Work out the finished part from the listing and answer in its coordinate system (mm). A direction names the side the tool comes from. Coordinates: 2 decimals unless noted, no trailing zeros. Order: outer loops, then holes, each group sorted by start corner. A loop starts at its lowest first (then second) coordinate and runs counter-clockwise, first axis right, second up. Notation, with made-up numbers: (82.5, -3) - (89.5, -3) arc R6 ccw to (89.5, 2) - close; hole circle Ø7 at (73, 37.25). An arc over 180 degrees is marked (long way). Answer as a JSON object with one key per item and string values. Group by question number.
1) Section B-B (y = 5) is taken. Give the vertices of the cut face in (x, z), plus the area to 3 significant figures.
2) Find the intervals of material crossed by line 1 along Z through (x, y) = (-10.45, 1.55); line 2 along X through (y, z) = (2.05, 5.2); line 3 along Z through (x, y) = (12.95, 2.55), in increasing order.
3) Section C-C (z = 5.2) is taken. Give the vertices of the cut face in (x, y).
4) Section A-A (x = -2.5) is taken. Give the vertices of the cut face in (y, z), plus the area to 3 significant figures.
5) The mould has two halves that part along Y. Classify faces 1 (the face through (1, 13, 14)), 2 (the face through (1, 9, -15)), 3 (the face through (-16.25, 1, 0)), 4 (the face through (-5.035, 5.535, 7.501)): released by +Y, released by -Y, zero draft, split by the parting line, or undercut.
6) Each of these flat-tipped pins is pushed along its axis until it touches: P1, Ø5, axis at x = -1, z = -14, coming from the -Y side; P2, Ø3.5, axis at x = -10.45, z = 15.6, coming from the +Y side; P3, Ø6, axis at x = -12.5, z = -1.5, coming from the +Y side. Where does it stop, or does it pass through?
7) Section D-D (y = 12) is taken. Give the vertices of the cut face in (x, z).
8) A tool of negligible diameter and unlimited length cuts with its end or side. For faces 5 (the face through (7.535, 5.465, 7.501)), 6 (the face through (6.965, 8.699, 14.69)), 7 (the face through (13.258, 2.081, -14.132)), 8 (the face through (1.32, 9.301, -7.485)), from which of +Z, -Z, +X, -X, +Y, -Y can it reach the whole face along a straight path? Write none if from no direction.
from build123d import *

# Parameters (mm, degrees)
SKETCH_2_W             = 32.5
SKETCH_2_H             = 42
SKETCH_2_R             = 1.5
SKETCH_2_R_2           = 1.449840903
EXTRUDE_1_DEPTH        = 3
SKETCH_4_W             = 12
SKETCH_4_H             = 42
CUT_EXTRUDE_1_DEPTH    = 22
EXTRUDE_2_DEPTH        = 42
FILLET_START           = 8
FILLET_1_OUTLINE_W     = 19
FILLET_1_OUTLINE_H     = 42
FILLET_1_DEPTH         = 5
FILLET_START_2         = -21
FILLET_1_2_DEPTH       = 42
FILLET_START_3         = 3
FILLET_1_3_OUTLINE_R   = 1.5
FILLET_1_3_OUTLINE_R_2 = 1.449840903
FILLET_1_3_DEPTH       = 5
CUT_EXTRUDE_2_REACH    = 31.565
SKETCH_6_W             = 36.57681216
SKETCH_6_H             = 14.4
FILLET_2_R             = 1


with BuildPart() as part:
    # Sketch 2 → Extrude 1 (new body)
    with BuildSketch(Plane(origin=(0, 0, 0), x_dir=(1, 0, 0), z_dir=(0, 1, 0))):
        Rectangle(SKETCH_2_W, SKETCH_2_H)
        with Locations(Location((-10.45, -15.6, 0), (0, 0, 270))):
            Circle(SKETCH_2_R, mode=Mode.SUBTRACT)
        with Locations(Location((-10.45, -5.2, 0), (0, 0, 270))):
            Circle(SKETCH_2_R, mode=Mode.SUBTRACT)
        with Locations(Location((-10.45, 5.2, 0), (0, 0, 270))):
            Circle(SKETCH_2_R, mode=Mode.SUBTRACT)
        with Locations(Location((-10.45, 15.6, 0), (0, 0, 270))):
            Circle(SKETCH_2_R, mode=Mode.SUBTRACT)
        with Locations(Location((12.95, 15.6, 0), (0, 0, 270))):
            Circle(SKETCH_2_R, mode=Mode.SUBTRACT)
        with Locations(Location((12.95, 5.2, 0), (0, 0, 270))):
            Circle(SKETCH_2_R, mode=Mode.SUBTRACT)
        with Locations(Location((12.899840903, -5.2, 0), (0, 0, 270))):
            Circle(SKETCH_2_R_2, mode=Mode.SUBTRACT)
        with Locations(Location((12.95, -15.6, 0), (0, 0, 270))):
            Circle(SKETCH_2_R, mode=Mode.SUBTRACT)
    extrude(amount=EXTRUDE_1_DEPTH)

    # Sketch 4 → Cut-Extrude 1 (cut)
    with BuildSketch(Plane(origin=(0, 3, 0), x_dir=(1, 0, 0), z_dir=(0, 1, 0))):
        with Locations((1.25, 0)):
            Rectangle(SKETCH_4_W, SKETCH_4_H)
    extrude(amount=-CUT_EXTRUDE_1_DEPTH, mode=Mode.SUBTRACT)


with BuildPart() as cut_extrude_1_piece_1:
    # of the separate pieces the step leaves, piece 1, a body of its own (cut_extrude_1_pieces)
    add(part.part.solids().sort_by_distance((-16.25, 0, 21))[0])



with BuildPart() as cut_extrude_1_piece_2:
    # of the separate pieces the step leaves, piece 2, a body of its own (cut_extrude_1_pieces)
    add(part.part.solids().sort_by_distance((7.25, 0, 21))[0])


with BuildPart() as cut_extrude_1_piece_1_1:
    add(cut_extrude_1_piece_1.part)

    add(cut_extrude_1_piece_2.part)  # Extrude 2 merges Cut-Extrude 1 piece 2
    # Sketch 5 → Extrude 2 (add)
    with BuildSketch(Plane.XY.offset(21)):
        Polygon((-4.75, 0), (-4.75, 3), (-4.75, 9), (7.25, 9), (7.25, 3), (7.25, 0), (10.75, 0), (10.75, 13), (-8.25, 13), (-8.25, 0), align=None)
    extrude(amount=-EXTRUDE_2_DEPTH)

    # Fillet 1: read off the stored shape, not the designer's step
    # Fillet 1 outline → Fillet 1 (cut)
    with BuildSketch(Plane(origin=(0, 0, 0), x_dir=(1, 0, 0), z_dir=(0, 1, 0)).offset(FILLET_START)):
        with Locations((1.25, 0)):
            Rectangle(FILLET_1_OUTLINE_W, FILLET_1_OUTLINE_H)
    extrude(amount=FILLET_1_DEPTH, mode=Mode.SUBTRACT)

    # Fillet 1 2 outline → Fillet 1 2 (add)
    with BuildSketch(Plane.XY.offset(FILLET_START_2)):
        with BuildLine():
            Line((-8.25, 3), (-8.25, 8))
            ThreePointArc((-8.25, 8), (-9.714466094, 4.464466094), (-13.25, 3))
            Line((-13.25, 3), (-8.25, 3))
        make_face()
        with BuildLine():
            ThreePointArc((15.75, 3), (12.214466094, 4.464466094), (10.75, 8))
            Line((10.75, 8), (10.75, 3))
            Line((10.75, 3), (15.75, 3))
        make_face()
        with BuildLine():
            Line((-4.75, 8), (-4.75, 9))
            Line((-4.75, 9), (7.25, 9))
            Line((7.25, 9), (7.25, 8))
            Line((7.25, 8), (10.75, 8))
            ThreePointArc((10.75, 8), (9.285533906, 11.535533906), (5.75, 13))
            Line((5.75, 13), (-3.25, 13))
            ThreePointArc((-3.25, 13), (-6.785533906, 11.535533906), (-8.25, 8))
            Line((-8.25, 8), (-4.75, 8))
        make_face()
    extrude(amount=FILLET_1_2_DEPTH)

    # Fillet 1 3 outline → Fillet 1 3 (cut)
    with BuildSketch(Plane(origin=(0, 0, 0), x_dir=(1, 0, 0), z_dir=(0, 1, 0)).offset(FILLET_START_3)):
        with Locations((-10.45, -15.6)):
            Circle(FILLET_1_3_OUTLINE_R)
        with Locations((-10.45, -5.2)):
            Circle(FILLET_1_3_OUTLINE_R)
        with Locations((-10.45, 5.2)):
            Circle(FILLET_1_3_OUTLINE_R)
        with Locations((-10.45, 15.6)):
            Circle(FILLET_1_3_OUTLINE_R)
        with Locations((12.899840903, -5.2)):
            Circle(FILLET_1_3_OUTLINE_R_2)
        with Locations((12.95, 15.6)):
            Circle(FILLET_1_3_OUTLINE_R)
        with Locations((12.95, 5.2)):
            Circle(FILLET_1_3_OUTLINE_R)
        with Locations((12.95, -15.6)):
            Circle(FILLET_1_3_OUTLINE_R)
    extrude(amount=FILLET_1_3_DEPTH, mode=Mode.SUBTRACT)

    # Cut-Extrude 2: up to this face of the body (flat: up to its plane)
    cut_extrude_2_end = Plane(cut_extrude_1_piece_1_1.part.faces().sort_by_distance((16, 3, 0))[0])
    # Sketch 6 → Cut-Extrude 2 (cut, up to the picked face)
    with BuildSketch(Plane(origin=(0, 13, 0), x_dir=(1, 0, 0), z_dir=(0, 1, 0)), mode=Mode.PRIVATE) as cut_extrude_2_sk1:
        Rectangle(SKETCH_6_W, SKETCH_6_H)
    cut_extrude_2_tool1 = split(extrude(cut_extrude_2_sk1.sketch, amount=-CUT_EXTRUDE_2_REACH, mode=Mode.PRIVATE), bisect_by=cut_extrude_2_end, keep=Keep.BOTH, mode=Mode.PRIVATE)
    add(cut_extrude_2_tool1.solids().sort_by(Axis((0, 13, 0), (0, -1, 0)))[0], mode=Mode.SUBTRACT)

    # Fillet 2
    fillet_2_edges = [cut_extrude_1_piece_1_1.edges().sort_by_distance(p)[0] for p in [
        (7.25, 9, 14.1),
        (-4.75, 9, 14.1),
        (-4.75, 6, -7.2),
        (1.25, 9, -7.2),
        (7.25, 6, -7.2),
        (-4.75, 6, 7.2),
        (7.25, 6, 7.2),
        (1.25, 9, 7.2),
        (-4.75, 9, -14.1),
        (7.25, 9, -14.1),
    ]]
    fillet(fillet_2_edges, radius=FILLET_2_R)


solid = cut_extrude_1_piece_1_1.part
Report:
{
 "1": {"outline": "(-9.25, -21) - (-4.75, -21) - (-4.75, -8.2) arc R1 ccw to (-5.75, -7.2) - (-9.25, -7.2) - (-9.25, -14.7) arc R1.5 cw to (-9.25, -16.5) - close; (-9.25, 7.2) - (-5.75, 7.2) arc R1 ccw to (-4.75, 8.2) - (-4.75, 21) - (-9.25, 21) - (-9.25, 16.5) arc R1.5 cw to (-9.25, 14.7) - close; (7.25, -21) - (11.75, -21) - (11.75, -16.5) arc R1.5 cw to (11.75, -14.7) - (11.75, -7.2) - (8.25, -7.2) arc R1 ccw to (7.25, -8.2) - close; (7.25, 8.2) arc R1 ccw to (8.25, 7.2) - (11.75, 7.2) - (11.75, 14.7) arc R1.5 cw to (11.75, 16.5) - (11.75, 21) - (7.25, 21) - close", "area": "246 mm²"},
 "2": {"line 1": "z = -21 to -17.1, -14.1 to -6.7, -3.7 to 3.7, 6.7 to 14.1, 17.1 to 21", "line 2": "x = -16.25 to -11.95, -8.95 to -4.75, 7.25 to 11.45, 14.35 to 16.25", "line 3": "z = -21 to -17.1, -14.1 to -6.7, -3.7 to 3.75, 6.65 to 14.1, 17.1 to 21"},
 "3": {"outline": "(-16.25, 0) - (-11.95, 0) - (-11.95, 3) - (-16.25, 3) - close; (-8.95, 0) - (-4.75, 0) - (-4.75, 3) - (-8.95, 3) - close; (7.25, 0) - (11.45, 0) - (11.45, 3) - (7.25, 3) - close; (14.35, 0) - (16.25, 0) - (16.25, 3) - (14.35, 3) - close"},
 "4": {"outline": "(9, -21) - (13, -21) - (13, -7.2) - (10, -7.2) arc R1 ccw to (9, -8.2) - close; (9, 8.2) arc R1 ccw to (10, 7.2) - (13, 7.2) - (13, 21) - (9, 21) - close", "area": "110 mm²"},
 "5": {"face 1": "released by +Y", "face 2": "released by -Y", "face 3": "zero draft", "face 4": "undercut"},
 "6": {"P1": "stops at y = 9", "P2": "stops at y = 5.93", "P3": "stops at y = 3"},
 "7": {"outline": "(-6.25, -21) - (8.75, -21) - (8.75, -7.2) - (-6.25, -7.2) - close; (-6.25, 7.2) - (8.75, 7.2) - (8.75, 21) - (-6.25, 21) - close"},
 "8": {"face 5": "none", "face 6": "+Z, -Z, -Y", "face 7": "+Y, -Y", "face 8": "-Y"}
}
